from build123d import *

# Parameters (mm, degrees)
SKETCH1_R           = 1.651
BOSS_EXTRUDE2_DEPTH = 3.175
BOSS_EXTRUDE3_DEPTH = 0.0254


with BuildPart() as part:
    # Sketch1 → Boss-Extrude2 (new body)
    with BuildSketch(Plane(origin=(0, 0, 0), x_dir=(1, 0, 0), z_dir=(0, 1, 0))):
        Polygon((0, -50.8), (-50.8, 0), (-71.12, 0), (-71.12, -10.16), (-10.16, -71.12), (0, -71.12), align=None)
        with Locations((-5.55625, -63.492108138)):
            Circle(SKETCH1_R, mode=Mode.SUBTRACT)
        with Locations((-11.90625, -50.8)):
            Circle(SKETCH1_R, mode=Mode.SUBTRACT)
        with Locations((-63.5, -5.42925)):
            Circle(SKETCH1_R, mode=Mode.SUBTRACT)
        with Locations((-50.8, -11.90625)):
            Circle(SKETCH1_R, mode=Mode.SUBTRACT)
    extrude(amount=BOSS_EXTRUDE2_DEPTH)

    # Sketch5 → Boss-Extrude3 (add)
    with BuildSketch(Plane(origin=(0, 3.175, 0), x_dir=(1, 0, 0), z_dir=(0, 1, 0))):
        Polygon((-28.185982934, -27.400888033), (-35.474882305, -27.400888033), (-32.595449328, -30.28032101), (-38.384718685, -36.069590367), (-36.729980154, -37.724328898), (-30.940710797, -31.935059541), (-28.185982934, -34.689787404), align=None)
    extrude(amount=BOSS_EXTRUDE3_DEPTH)


solid = part.part
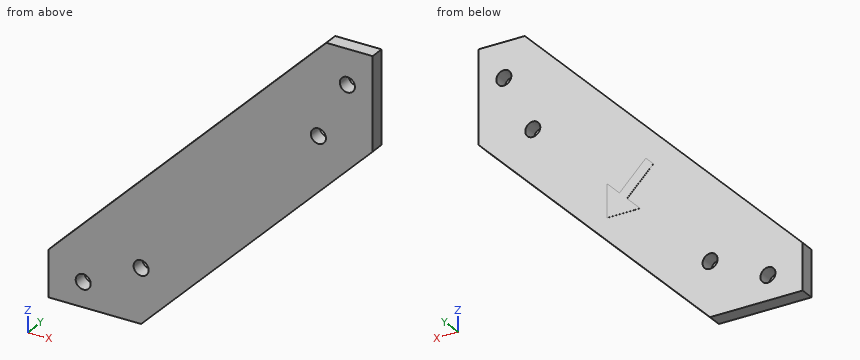
Could you check a few things on this model? Use its own coordinates, in mm. Coordinates: 2 decimals unless noted, no trailing zeros. Order: outer loops, then holes, each group sorted by start corner. A loop starts at its lowest first (then second) coordinate and runs counter-clockwise, first axis right, second up.
Q1. Suppose I cut it at A-A on x = -63.5. Please give me the cut outline in (y, z) (3 decimals), and give its area (3 significant figures).
Q2. Will these pins go through, and if not, where does the flat tip stop? pin 1 (1.5 mm diameter, centred on y = 3, z = 57.5, fed in from -X); pin 2 (1 mm diameter, centred on x = -30.5, y = 1.5, fed in from -Z); pin 3 (4 mm diameter, centred on x = -63.5, z = 5.43, fed in from +Y) (3 decimals).
Q3. Suppose I cut it at C-C on x = -20. Please give me the cut outline in (y, z) (3 decimals), and give its area (3 significant figures).
Q4. Suppose I cut it at B-B on y = 0.85. Please give me the cut outline in (x, z), and give its area (3 significant figures).
Q5. Suppose I cut it at D-D on z = 46.5. Please give me the cut outline in (x, y) (3 decimals).
Q6. Please list where these lines run through material, in increasing order: L1, parallel to Y at x = -46, z = 7 (3 decimals); L2, parallel to Z at x = -63.5, y = 2.35; L3, parallel to Z at x = -7, y = 2.85.
Answer:
1. outline: (0, 0) - (3.175, 0) - (3.175, 3.778) - (0, 3.778) - close; (0, 7.08) - (3.175, 7.08) - (3.175, 17.78) - (0, 17.78) - close
1. area: 46.0 mm2
2. pin 1: stops at x = -24.53
2. pin 2: stops at z = 19.8
2. pin 3: stops at y = 3.175
3. outline: (0, 30.8) - (3.175, 30.8) - (3.175, 61.28) - (0, 61.28) - close
3. area: 96.8 mm2
4. outline: (-71.12, 0) - (-50.8, 0) - (0, 50.8) - (0, 71.12) - (-10.16, 71.12) - (-71.12, 10.16) - close; hole circle Ø3.3 at (-63.5, 5.43); hole circle Ø3.3 at (-50.8, 11.91); hole circle Ø3.3 at (-11.91, 50.8); hole circle Ø3.3 at (-5.56, 63.49)
4. area: 1,880 mm2
5. outline: (-34.78, 0) - (-4.3, 0) - (-4.3, 3.175) - (-34.78, 3.175) - close
6. L1: y = 0 to 3.175
6. L2: z = 0 to 3.78, 7.08 to 17.78
6. L3: z = 43.8 to 62.69, 64.29 to 71.12
